Here's how the part is built. I have some questions about the finished solid (model axes, mm). Face numbers are marked on the shaded views. A direction names the side the tool comes from. Coordinates: 2 decimals unless noted, no trailing zeros. Write each loop counter-clockwise with the first axis right and the second up, starting at its lowest first coordinate (ties: lowest second). Pieces come first, ordered by that corner, then holes.
(1) Please list where these lines run through material, in increasing order: probe 1 along X at (y, z) = (0, 1.65); probe 2 along Y at (x, z) = (-0.25, 1.35); probe 3 along Y at (x, z) = (0, 1.9).
(2) Which directions (+Z, -Z, +X, -X, +Y, -Y) give clear straight access to the entire face, cutting with the end or side of a thin tool? Please do the marked faces 1, 2, 3 and 4.
(3) Imagine slicing it at A-A, the plane y = 0. List the corners of the cut face in (x, z) for me.
(4) Imagine slicing it at C-C, the plane z = 0.2. List the corners of the cut face in (x, y) for me, plus the area to 3 significant figures.
(5) Thinking about a two-plate mould opening in Y: for the marked faces 5, 6, 7 and 8, which applies, released by +Y, released by -Y, zero draft, split by the parting line, or undercut?
Autodesk Fusion 360 part; units mm, degrees
sketch "Sketch1" plane through (0, 0, 0) normal (0, 0, 1) x (1, 0, 0)
  line L0 (4, 2.7) -> (-4, 2.7)
  line L1 (-4, 2.7) -> (-4, -2.7)
  line L2 (-4, -2.7) -> (4, -2.7)
  line L3 (4, -2.7) -> (4, 2.7)
  line L4 (4, 2.7) -> (-4, -2.7) construction
  line L5 (-4, 2.7) -> (4, -2.7) construction
  circle A0 centre (0, 0) radius 1.5
  dimension "d1" = 5.4
  dimension "d2" = 8
  dimension "d3" = 3
extrude "Extrude1" add sketch "Sketch1" along normal blind 2.4
fillet "Fillet1" radius 2 2 edges at (0, -2.7, 2.4) (0, 2.7, 2.4)
chamfer "Chamfer2" distance 1.4 distance2 1.4 1 edges at (-4, 0, 0) measured on face at (-4, 0.2333, 0.8)
sketch "Sketch2" plane through (0, 0, 0) normal (0, 0, -1) x (1, 0, 0)
  line L0 (-2.6, 2.7) -> (-2.6, -2.7)
  line L1 (-2.6, -2.7) -> (4, -2.7)
  line L2 (4, -2.7) -> (4, 2.7)
  line L3 (4, 2.7) -> (-2.6, 2.7)
  circle A0 centre (0, 0) radius 1.5
  line L4 (0, 2.7) -> (0, -2.7) construction
  line L5 (2.7, -2.7) -> (2.7, 2.7)
  dimension "d12" = 2.7
chamfer "Chamfer3" distance 0.4 angle 45 4 edges at (0.7, -2.7, 0) (4, 0, 0) (0.7, 2.7, 0) (-1.3985, 0.5424, 0)
equation "d12 = ( 5.4 / 2 ) * 1 mm"
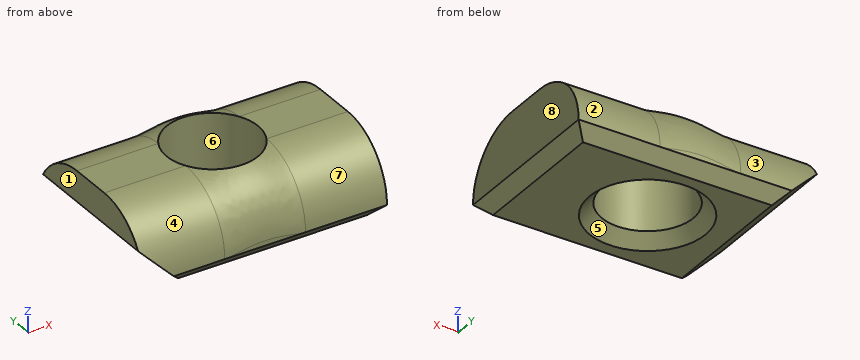
Recorded:
1. probe 1: x = -4 to -1.5, 1.5 to 4
1. probe 2: y = -2.54 to -1.48, 1.48 to 2.54
1. probe 3: y = -2.19 to -1.5, 1.5 to 2.19
2. face 1: +Z, -Z, -X, +Y, -Y
2. face 2: +Z, +X, +Y
2. face 3: +Z, -X, +Y
2. face 4: +Z, -X, -Y
3. outline: (-4, 1.4) - (-2.6, 0) - (-1.9, 0) - (-1.5, 0.4) - (-1.5, 2.4) - (-4, 2.4) - close; (1.5, 0.4) - (1.9, 0) - (3.6, 0) - (4, 0.4) - (4, 2.4) - (1.5, 2.4) - close
4. outline: (-2.8, -2.5) - (3.8, -2.5) - (3.8, 2.5) - (-2.8, 2.5) - close; hole circle Ø3.4 at (0, 0)
4. area: 23.9 mm2
5. face 5: undercut
5. face 6: undercut
5. face 7: released by -Y
5. face 8: zero draft
